Model file for the job. Use its own axes, mm. Round coordinates to 2 decimals unless told otherwise and drop trailing zeros. Order: outer loops, then holes, each group sorted by start corner. A loop starts at its lowest first (then second) coordinate and runs counter-clockwise, first axis right, second up. Notation, with made-up numbers: (-40, -9.75) -> (17, -9.75) arc R24 cw to (17, 18.25) -> close; hole circle Ø1 at (22, 5). An arc over 180 degrees is marked (long way). Put each result on its own line as item: value. Start each with the question number.
Q1. Probe L1, parallel to X at y = 21, z = 0.5; L2, parallel to X at y = 0.5, z = 2; L3, parallel to Y at x = -9, z = 1.5. List the from-to ranges inside material, lowest first.
Q2. Cut at C-C, the plane x = -13. State how many separate pieces and enclosed holes the cut face has, and give its area (3 significant figures).
Q3. Cut at A-A, the plane x = 58. List the corners of the cut face in (y, z).
Q4. Cut at B-B, the plane y = -11.5. List the corners of the cut face in (x, z), and give its area (3 significant figures).
Q5. Flat gauge pins, fed straight in: P1, Ø1.1, axis at x = -33, z = 1.5, coming from the +Y side; P2, Ø1.5, axis at y = 7, z = 2.5, coming from the -X side. Where does each tip first touch, or does it go through?
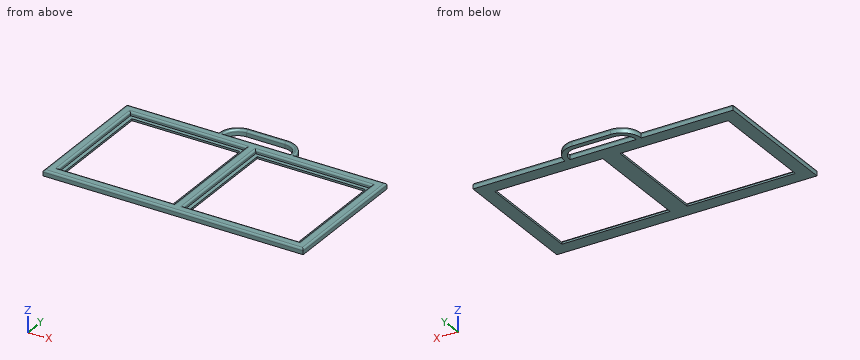
from build123d import *

# Parameters (mm, degrees)
F0_W     = 2.5711264648
F0_H     = 5
F1_DEPTH = 3
F0_W_2   = 56.75
F0_H_2   = 56.75
F2_DEPTH = 1
F3_R     = 1


# Not quite as in the source:
# - a feature names something its author has since deleted; it is built from what else it names


with BuildPart() as f1:
    # F0 (on Top) → F1 (new body)
    with BuildSketch(Plane.XY):
        Polygon((-63.25, -34.2033516131), (-63.25, 26.5466483869), (-20, 26.5466483869), (-20, 31.5466483869), (-34.125, 31.5466483869), (-68.25, 31.5466483869), (-68.25, -39.2033516131), (0, -39.2033516131), (0, 31.5466483869), (-17.4288735352, 31.5466483869), (-17.4288735352, 26.5466483869), (-2.5, 26.5466483869), (-2.5, -34.2033516131), align=None)
        with Locations((-18.7144367676, 29.0466483869)):
            Rectangle(F0_W, F0_H)
        with BuildLine():
            ThreePointArc((-10, 41.5466483869), (-17.0710678119, 38.6177161988), (-20, 31.5466483869))
            Line((-20, 31.5466483869), (-17.4288735352, 31.5466483869))
            ThreePointArc((-17.4288735352, 31.5466483869), (-15.2530068533, 36.7996552402), (-10, 38.9755219221))
            Line((-10, 38.9755219221), (0, 38.9755219221))
            Line((0, 38.9755219221), (0, 41.5466483869))
            Line((0, 41.5466483869), (-10, 41.5466483869))
        make_face()
    extrude(amount=F1_DEPTH)

    # F0 (on Top) → F2 (join)
    with BuildSketch(Plane.XY):
        Polygon((-20, 26.5466483869), (-63.25, 26.5466483869), (-63.25, -34.2033516131), (-2.5, -34.2033516131), (-2.5, 26.5466483869), (-17.4288735352, 26.5466483869), align=None)
        with Locations((-32.875, -3.8283516131)):
            Rectangle(F0_W_2, F0_H_2, mode=Mode.SUBTRACT)
    extrude(amount=F2_DEPTH)

    # F3
    f3_edges = [f1.edges().sort_by_distance(p)[0] for p in [
        (-32.875, 26.546648, 3),
        (-63.25, -3.828352, 3),
        (-32.875, -34.203352, 3),
        (-2.5, -3.828352, 3),
        (-68.25, -3.828352, 3),
        (-34.125, -39.203352, 3),
        (-8.714437, 31.546648, 3),
        (-15.253007, 36.799655, 3),
        (-17.071068, 38.617716, 3),
        (-5, 38.975522, 3),
        (-5, 41.546648, 3),
        (-44.125, 31.546648, 3),
    ]]
    fillet(f3_edges, radius=F3_R)

    # F4: F1 across plane


with BuildPart() as f1_1:
    add(f1.part)
    add(f1.part.mirror(Plane.YZ))


solid = f1_1.part
Ans:
1. L1: x = -68.25 to -61.25, -4.5 to 4.5, 61.25 to 68.25
1. L2: x = -68.25 to -63.25, -2.5 to 2.5, 63.25 to 68.25
1. L3: y = -39.2 to -34.2, 26.55 to 31.55, 38.98 to 41.55
2. separate pieces: 3
2. enclosed holes: 0
2. area: 40.9 mm^2
3. outline: (-39.2, 0) -> (-32.2, 0) -> (-32.2, 1) -> (-34.2, 1) -> (-34.2, 2) arc R1 ccw to (-35.2, 3) -> (-38.2, 3) arc R1 ccw to (-39.2, 2) -> close; (24.55, 0) -> (31.55, 0) -> (31.55, 2) arc R1 ccw to (30.55, 3) -> (27.55, 3) arc R1 ccw to (26.55, 2) -> (26.55, 1) -> (24.55, 1) -> close
4. outline: (-68.25, 0) -> (-61.25, 0) -> (-61.25, 1) -> (-63.25, 1) -> (-63.25, 2) arc R1 ccw to (-64.25, 3) -> (-67.25, 3) arc R1 ccw to (-68.25, 2) -> close; (-4.5, 0) -> (4.5, 0) -> (4.5, 1) -> (2.5, 1) -> (2.5, 2) arc R1 ccw to (1.5, 3) -> (-1.5, 3) arc R1 ccw to (-2.5, 2) -> (-2.5, 1) -> (-4.5, 1) -> close; (61.25, 0) -> (68.25, 0) -> (68.25, 2) arc R1 ccw to (67.25, 3) -> (64.25, 3) arc R1 ccw to (63.25, 2) -> (63.25, 1) -> (61.25, 1) -> close
4. area: 51.7 mm^2
5. P1: stops at y = 31.55
5. P2: stops at x = -68.25
